from build123d import *

# Parameters (mm, degrees)
SKETCH1_R           = 6
BOSS_EXTRUDE1_DEPTH = 20
BOSS_EXTRUDE2_START = 1
SKETCH2_W           = 15
SKETCH2_H           = 20
BOSS_EXTRUDE2_DEPTH = 5
SKETCH3_R           = 3.1
CUT_EXTRUDE1_DEPTH  = 23.186707732
BOSS_EXTRUDE3_START = -6
BOSS_EXTRUDE3_DEPTH = 6
SKETCH5_R           = 0.5
CUT_EXTRUDE2_DEPTH  = 10
SKETCH6_W           = 15
SKETCH6_H           = 20
BOSS_EXTRUDE4_DEPTH = 8
SKETCH7_W           = 30
SKETCH7_H           = 30
BOSS_EXTRUDE5_DEPTH = 2
FILLET1_R           = 3


with BuildPart() as part:
    # Sketch1 → Boss-Extrude1 (new body)
    with BuildSketch(Plane.XY):
        Circle(SKETCH1_R)
    extrude(amount=BOSS_EXTRUDE1_DEPTH)

    # Sketch2 → Boss-Extrude2 (add)
    with BuildSketch(Plane(origin=(0, 0, 0), x_dir=(1, 0, 0), z_dir=(0, 1, 0)).offset(BOSS_EXTRUDE2_START)):
        with Locations((0, -10)):
            Rectangle(SKETCH2_W, SKETCH2_H)
    extrude(amount=BOSS_EXTRUDE2_DEPTH)

    # Sketch3 → Cut-Extrude1 (cut, through all)
    with BuildSketch(Plane(origin=(0, 0, 0), x_dir=(-1, 0, 0), z_dir=(0, 0, -1))):
        Circle(SKETCH3_R)
    extrude(amount=-CUT_EXTRUDE1_DEPTH, mode=Mode.SUBTRACT)

    # Sketch4 → Boss-Extrude3 (add)
    with BuildSketch(Plane.XY.offset(20).offset(BOSS_EXTRUDE3_START)):
        with BuildLine():
            ThreePointArc((5.916079783, 1), (5.977725364, -0.516526349), (5.656854249, -2))
            Line((5.656854249, -2), (7.5, -2))
            Line((7.5, -2), (7.5, 1))
            Line((7.5, 1), (5.916079783, 1))
        make_face()
        with BuildLine():
            Line((-7.5, -2), (-5.656854249, -2))
            ThreePointArc((-5.656854249, -2), (-5.977725364, -0.516526349), (-5.916079783, 1))
            Line((-5.916079783, 1), (-7.5, 1))
            Line((-7.5, 1), (-7.5, -2))
        make_face()
    extrude(amount=BOSS_EXTRUDE3_DEPTH)

    # Sketch5 → Cut-Extrude2 (cut)
    with BuildSketch(Plane.XY.offset(20)):
        with Locations((-6.341942864, -0.319782293)):
            Circle(SKETCH5_R)
        with Locations((-4.344480544, -0.219063461)):
            Circle(SKETCH5_R)
        with Locations((4.94371924, 0.249279111)):
            Circle(SKETCH5_R)
        with Locations((6.860426101, 0.249279111)):
            Circle(SKETCH5_R)
    extrude(amount=-CUT_EXTRUDE2_DEPTH, mode=Mode.SUBTRACT)

    # Sketch6 → Boss-Extrude4 (add)
    with BuildSketch(Plane(origin=(0, 6, 0), x_dir=(1, 0, 0), z_dir=(0, 1, 0))):
        with Locations((0, -10)):
            Rectangle(SKETCH6_W, SKETCH6_H)
    extrude(amount=BOSS_EXTRUDE4_DEPTH)

    # Sketch7 → Boss-Extrude5 (add)
    with BuildSketch(Plane(origin=(0, 14, 0), x_dir=(1, 0, 0), z_dir=(0, 1, 0))):
        with Locations((0, -10)):
            Rectangle(SKETCH7_W, SKETCH7_H)
    extrude(amount=BOSS_EXTRUDE5_DEPTH)

    # Fillet1
    fillet1_edges = [part.edges().sort_by_distance(p)[0] for p in [
        (0, 14, 0),
        (-7.5, 14, 10),
        (0, 14, 20),
        (7.5, 14, 10),
    ]]
    fillet(fillet1_edges, radius=FILLET1_R)


solid = part.part
Can you work these out from the model? Positions are in its coordinate system, mm. A direction names the side the tool comes from. Round coordinates to 2 decimals unless told otherwise and drop trailing zeros. Loops run counter-clockwise (first coordinate to the right, second up) from the corner with the lowest first, then second, coordinate; pieces in that order, holes last. Notation, with made-up numbers: (78, 22.5) - (115, 22.5) arc R27 ccw to (115, 57.5) - close; hole circle Ø6 at (32, 77). An arc over 180 degrees is marked (long way). Use CSV: the item, a comma, the result in double quotes. Start each with the question number.
1) For faces 4 (the flat face through (0, 4, 0)), 5 (the flat face through (0, 4, 20)), 6 (the cylindrical face through (-5.865, -0.17, 16.181)), 7 (the flat face through (7, -2, 17)), 8 (the flat face through (-7, -2, 17)), which set-ups out of +Z, -Z, +X, -X, +Y, -Y let a thin tool reach every point of the face, with its end or its side?
2) We'd pull the mould along X, two halves only. Please class faces 1 (the cylindrical face through (0.15, 13.14, 20.9)), 2 (the flat face through (-4.4, -0.2, 10)), 3 (the flat face through (7.5, 6, 10)): released by +X, released by -X, zero draft, split by the parting line, or undercut.
3) If we section it at A-A on x = 0: Write out the boundary of the cut face in (y, z).
4) If we section it at D-D on y = 3.5: Write out the boundary of the cut face in (x, z), plus the area to 3 significant figures.
5) If we section it at B-B on z = 3.75: Write out the boundary of the cut face in (x, y), plus the area to 3 significant figures.
6) If we section it at C-C on z = -0.5: Write out the boundary of the cut face in (x, y), plus the area to 3 significant figures.
7) For pin 1 Ø2 at (x, z) = (-6.5, 18) entering from -Y; pin 2 Ø1.5 at (x, y) = (6, 0) entering from -Z; pin 3 Ø12 at (y, z) = (-3, -2) entering from +X, each with a flat end and sliding along its axis, tell me the tip position at first contact or that it passes through.
8) Please list where these lines run through material, in increasing order: probe 1 along X at (y, z) = (0.25, 6.5); probe 2 along Y at (x, z) = (0, 5.75); probe 3 along X at (y, z) = (10.75, 2). Write a range as [from, to].
Geometry results:
1,face 4,"-Z, +X, -X, -Y"
1,face 5,"+Z, +X, -X, -Y"
1,face 6,"+Z"
1,face 7,"+Z, -Z, +X, -Y"
1,face 8,"+Z, -Z, -X, -Y"
2,face 1,"zero draft"
2,face 2,"undercut"
2,face 3,"released by +X"
3,outline,"(-6, 0) - (-3.1, 0) - (-3.1, 20) - (-6, 20) - close; (3.1, 0) - (11, 0) arc R3 cw to (14, -3) - (14, -5) - (16, -5) - (16, 25) - (14, 25) - (14, 23) arc R3 cw to (11, 20) - (3.1, 20) - close"
4,outline,"(-7.5, 0) - (7.5, 0) - (7.5, 20) - (-7.5, 20) - close"
4,area,"300 mm2"
5,outline,"(-15, 14) - (-10.5, 14) arc R3 cw to (-7.5, 11) - (-7.5, 1) - (-5.92, 1) arc R6 ccw (long way) to (5.92, 1) - (7.5, 1) - (7.5, 11) arc R3 cw to (10.5, 14) - (15, 14) - (15, 16) - (-15, 16) - close; hole circle Ø6.2 at (0, 0)"
5,area,"297 mm2"
6,outline,"(-15, 14) - (-10.5, 14) arc R3 cw to (-8, 12.66) - (8, 12.66) arc R3 cw to (10.5, 14) - (15, 14) - (15, 16) - (-15, 16) - close"
6,area,"83.5 mm2"
7,pin 1,"stops at y = -2.4"
7,pin 2,"stops at z = 0"
7,pin 3,"stops at x = 7.5"
8,probe 1,"x = [-5.99, -3.09], [3.09, 5.99]"
8,probe 2,"y = [-6, -3.1], [3.1, 16]"
8,probe 3,"x = [-7.5, 7.5]"
